from build123d import *

# Parameters (mm, degrees)
SKETCH3_W                 = 60.96
SKETCH3_H                 = 60.96
BOSS_EXTRUDE1_DEPTH       = 3.175
F_6_0_15_DIAMETER_HOLE1_D = 3.81
SKETCH6_W                 = 60.96
SKETCH6_H                 = 3.175
BOSS_EXTRUDE3_DEPTH       = 30.48
F_6_0_15_DIAMETER_HOLE2_D = 3.81


with BuildPart() as part:
    # Sketch3 → Boss-Extrude1 (new body)
    with BuildSketch(Plane(origin=(0, 0, 0), x_dir=(1, 0, 0), z_dir=(0, 1, 0))):
        with Locations((30.48, 30.48)):
            Rectangle(SKETCH3_W, SKETCH3_H)
    extrude(amount=BOSS_EXTRUDE1_DEPTH)

    # #6 (0.15) Diameter Hole1 (through all)
    with Locations(Plane(origin=(0, 3.175, 0), x_dir=(1, 0, 0), z_dir=(0, 1, 0))):
        with Locations((15.24, 15.24), (45.72, 15.24)):
            Hole(F_6_0_15_DIAMETER_HOLE1_D / 2)

    # Sketch6 → Boss-Extrude3 (add)
    with BuildSketch(Plane.XZ):
        with Locations((30.48, -1.5875)):
            Rectangle(SKETCH6_W, SKETCH6_H)
    extrude(amount=BOSS_EXTRUDE3_DEPTH)

    # #6 (0.15) Diameter Hole2 (through all)
    with Locations(Plane.XY):
        with Locations((15.24, -12.065), (45.72, -12.065)):
            Hole(F_6_0_15_DIAMETER_HOLE2_D / 2)


solid = part.part
Model file for the job. Use its own axes, mm. A direction names the side the tool comes from. Give positions to 0.01 mm unless a question says otherwise; leave off trailing zeros. Loops run counter-clockwise (first coordinate to the right, second up) from the corner with the lowest first, then second, coordinate; pieces in that order, holes last. Notation, with made-up numbers: (-5, -19) -> (17, -19) arc R29 cw to (17, 8) -> close; hole circle Ø3 at (27.25, 28). An arc over 180 degrees is marked (long way). Use a Markdown table: item, result. Add a question column.
(1) Tool access for faces 1 (the cylindrical face through (46.13, 1.57, -13.38)), 2 (the flat face through (30, -15, -3.175)): list every direction of +Z, -Z, +X, -X, +Y, -Y with a clear straight run to the whole face (end or side of a thin tool).
(2) Slice it at C-C on x = 28. List the corners of the cut face in (y, z) (3 decimals), and give its area (3 significant figures).
(3) Slice it at B-B on z = -15.24. List the corners of the cut face in (x, y) (3 decimals), and give its area (3 significant figures).
(4) Wall check: line 1 along X through (y, z) = (1.7, -15.24) (3 decimals); line 2 along Z through (x, y) = (15, 1); line 3 along Y through (x, z) = (15.24, -1.8) (3 decimals). Give the ranges that are in metal, low to high.
(5) Slice it at A-A on x = 45.72. List the corners of the cut face in (y, z) (3 decimals).
(6) Mould opens along Y. For faces 3 (the flat face through (60.96, 1, -24)), 4 (the cylindrical face through (15.653, -13.925, -1.61)), 5 (the flat face through (30, -30.48, -2)) say: +Y half, -Y half, draft (parallel to the pull), parting line (faces both ways), or undercut.
(7) Drop flat-ended pins along their axis: pin 1 Ø6 at (x, z) = (45.72, -15.24) entering from -Y; pin 2 Ø1.5 at (x, y) = (28, -3.5) entering from -Z (3 decimals). Give the stop position or say it passes through.
(8) Slice it at D-D on y = -15.5. List the corners of the cut face in (x, z) (3 decimals).
Filled sheet:
| question | item | result |
|---|---|---|
| 1 | face 1 | +Y, -Y |
| 1 | face 2 | -Z, +X, -X, -Y |
| 2 | outline | (-30.48, -3.175) -> (0, -3.175) -> (0, -60.96) -> (3.175, -60.96) -> (3.175, 0) -> (-30.48, 0) -> close |
| 2 | area | 290 mm2 |
| 3 | outline | (0, 0) -> (13.335, 0) -> (13.335, 3.175) -> (0, 3.175) -> close; (17.145, 0) -> (43.815, 0) -> (43.815, 3.175) -> (17.145, 3.175) -> close; (47.625, 0) -> (60.96, 0) -> (60.96, 3.175) -> (47.625, 3.175) -> close |
| 3 | area | 169 mm2 |
| 4 | line 1 | 0 to 13.335, 17.145 to 43.815, 47.625 to 60.96 |
| 4 | line 2 | -60.96 to -17.13, -13.35 to 0 |
| 4 | line 3 | -30.48 to -13.97, -10.16 to 3.175 |
| 5 | outline | (-30.48, -3.175) -> (-13.97, -3.175) -> (-13.97, 0) -> (-30.48, 0) -> close; (-10.16, -3.175) -> (0, -3.175) -> (0, -13.335) -> (3.175, -13.335) -> (3.175, 0) -> (-10.16, 0) -> close; (0, -60.96) -> (3.175, -60.96) -> (3.175, -17.145) -> (0, -17.145) -> close |
| 6 | face 3 | draft |
| 6 | face 4 | undercut |
| 6 | face 5 | -Y half |
| 7 | pin 1 | y = 0 |
| 7 | pin 2 | z = -3.175 |
| 8 | outline | (0, -3.175) -> (60.96, -3.175) -> (60.96, 0) -> (0, 0) -> close |
